```python
from build123d import *

# Parameters (mm, degrees)
F1_DEPTH = 5
F4_DEPTH = 2.54
F5_DEPTH = 25.4


with BuildPart() as f1:
    # F0 (on Front) → F1 (new body)
    with BuildSketch(Plane.XZ):
        with BuildLine():
            ThreePointArc((0, 20.9869445181), (-12.0966427586, 25.9236544676), (-24.1932855172, 20.9869445181))
            ThreePointArc((-24.1932855172, 20.9869445181), (-32.8877742223, 9.0834832543), (-21.2784307494, 0))
            ThreePointArc((-21.2784307494, 0), (-27.8345018972, -12.2317448258), (-21.2784307494, -24.4634896517))
            ThreePointArc((-21.2784307494, -24.4634896517), (-35.1701421662, -37.2707710413), (-38.4840406477, -55.8724962175))
            ThreePointArc((-38.4840406477, -55.8724962175), (-23.8469055846, -52.8720513548), (-9.2097705214, -55.8724962175))
            ThreePointArc((-9.2097705214, -55.8724962175), (-6.0029489911, -61.8966557159), (-2.7961274609, -55.8724962175))
            ThreePointArc((-2.7961274609, -55.8724962175), (9.7817579313, -54.6124723986), (22.2429726273, -56.7359104753))
            ThreePointArc((22.2429726273, -56.7359104753), (22.2759376745, -54.9746026101), (22.22623583, -53.2136875591))
            ThreePointArc((22.22623583, -53.2136875591), (18.366243738, -38.4713383456), (8.9641526372, -26.4781285077))
            ThreePointArc((8.9641526372, -26.4781285077), (9.8457214763, -18.7313808571), (8.9641526372, -10.9846332065))
            ThreePointArc((8.9641526372, -10.9846332065), (12.7377833841, 3.0446666193), (5.6262267365, 15.7130250237))
            Line((5.6262267365, 15.7130250237), (36.5616049228, 40.8807976003))
            ThreePointArc((36.5616049228, 40.8807976003), (34.4898748978, 53.7428757551), (23.25864156, 47.1410186325))
            Line((23.25864156, 47.1410186325), (0, 20.9869445181))
        make_face()
    extrude(amount=F1_DEPTH)

    # F5 (cut): a face of the model
    f5_faces = [f1.faces().sort_by_distance(p)[0] for p in [
        (-4.5967380367, -5, -11.98241047),
    ]]
    extrude(f5_faces, amount=-F5_DEPTH, mode=Mode.SUBTRACT)


with BuildPart() as f1b:
    # F0 (on Front) → F1, piece 2 (new body)
    with BuildSketch(Plane.XZ):
        with BuildLine():
            ThreePointArc((41.8436169818, -52.7066290379), (31.7747593943, -42.8946624715), (22.22623583, -53.2136875591))
            ThreePointArc((22.22623583, -53.2136875591), (32.2819872673, -62.5185956042), (41.8436169818, -52.7066290379))
        make_face()
    extrude(amount=F1_DEPTH)


with BuildPart() as f4:
    # F3 (on face) → F4 (new body)
    with BuildSketch(Plane.XZ.offset(5)):
        with BuildLine():
            ThreePointArc((-40.3169446951, -59.5749264298), (-26.5786982557, -55.5198668281), (-12.3739342893, -57.3658365623))
            ThreePointArc((-12.3739342893, -57.3658365623), (-6.2221601499, -64.4329037682), (0.3986158134, -57.8031911351))
            ThreePointArc((0.3986158134, -57.8031911351), (12.6136445695, -57.3475459696), (24.4946623983, -60.2208638043))
            ThreePointArc((24.4946623983, -60.2208638043), (22.3566756727, -41.3285471938), (11.7528280148, -25.5472598891))
            ThreePointArc((11.7528280148, -25.5472598891), (12.3852570181, -18.5459373039), (11.6827134618, -11.5513024358))
            ThreePointArc((11.6827134618, -11.5513024358), (15.3563975367, 2.4028081974), (9.5009837393, 15.5909577077))
            Line((9.5009837393, 15.5909577077), (38.2345170044, 38.9673983055))
            ThreePointArc((38.2345170044, 38.9673983055), (36.0298866682, 55.8114240261), (20.82786015, 48.229868306))
            Line((20.82786015, 48.229868306), (-0.2458838852, 24.5326862524))
            ThreePointArc((-0.2458838852, 24.5326862524), (-13.043561552, 28.4410317154), (-25.4100113891, 23.3296095701))
            ThreePointArc((-25.4100113891, 23.3296095701), (-35.5065684593, 11.3015480777), (-26.8662872673, -1.811814148))
            ThreePointArc((-26.8662872673, -1.811814148), (-30.3536378615, -13.0793756448), (-25.7757993219, -23.9496539557))
            ThreePointArc((-25.7757993219, -23.9496539557), (-38.9666786297, -39.3458023105), (-40.3169446951, -59.5749264298))
        make_face()
        with BuildLine():
            ThreePointArc((-2.7961274609, -55.8724962175), (-6.0029489911, -61.8966557159), (-9.2097705214, -55.8724962175))
            ThreePointArc((-9.2097705214, -55.8724962175), (-23.8469055846, -52.8720513548), (-38.4840406477, -55.8724962175))
            ThreePointArc((-38.4840406477, -55.8724962175), (-35.1701421662, -37.2707710413), (-21.2784307494, -24.4634896517))
            ThreePointArc((-21.2784307494, -24.4634896517), (-27.8345018972, -12.2317448258), (-21.2784307494, 0))
            ThreePointArc((-21.2784307494, 0), (-32.8877742223, 9.0834832543), (-24.1932855172, 20.9869445181))
            ThreePointArc((-24.1932855172, 20.9869445181), (-12.0966427586, 25.9236544676), (0, 20.9869445181))
            Line((0, 20.9869445181), (23.25864156, 47.1410186325))
            ThreePointArc((23.25864156, 47.1410186325), (34.4898748978, 53.7428757551), (36.5616049228, 40.8807976003))
            Line((36.5616049228, 40.8807976003), (5.6262267365, 15.7130250237))
            ThreePointArc((5.6262267365, 15.7130250237), (12.7377833841, 3.0446666193), (8.9641526372, -10.9846332065))
            ThreePointArc((8.9641526372, -10.9846332065), (9.8457214763, -18.7313808571), (8.9641526372, -26.4781285077))
            ThreePointArc((8.9641526372, -26.4781285077), (19.1118233272, -40.0673969806), (22.2429726273, -56.7359104753))
            ThreePointArc((22.2429726273, -56.7359104753), (9.7817579313, -54.6124723986), (-2.7961274609, -55.8724962175))
        make_face(mode=Mode.SUBTRACT)
    extrude(amount=F4_DEPTH)


solid = f4.part
```
Can you work these out from the model? Positions are in its coordinate system, mm. A direction names the side the tool comes from. Coordinates: 2 decimals unless noted, no trailing zeros. Order: outer loops, then holes, each group sorted by start corner. A loop starts at its lowest first (then second) coordinate and runs counter-clockwise, first axis right, second up.
1. Thinking about a two-plate mould opening in Z: for faces 3 (the face through (9.846, -6.252, -18.622)), 4 (the face through (12.44, -6.25, -57.33)), 5 (the face through (10.44, -6.25, 36.55)), 6 (the face through (12, -5, -8)), which applies, +Z half, -Z half, draft (parallel to the pull), parting line (faces both ways), or undercut?
2. If we section it at C-C (x = 19): Please give me the cut outline in (y, z), then the cut area to 3 significant figures.
3. I'm going to push flat-ended pins straight in: pin 1 (1 mm diameter, centred on y = -5.5, z = -27.5, fed in from +X); pin 2 (1 mm diameter, centred on x = -8.5, y = -5.5, fed in from -Z); pin 3 (1.5 mm diameter, centred on x = -24.5, y = -7, fed in from -Z). Where does each tip first touch, or does it pass through?
4. For faces 1 (the face through (-26.78, -6.252, -55.536)), 2 (the face through (-12.284, -6.252, 25.923)), which set-ups out of +Z, -Z, +X, -X, +Y, -Y let a thin tool reach every point of the face, with its end or its side?
5. If we section it at D-D (y = -5.5): Please give me the cut outline in (x, z), then the cut area to 3 significant figures.
6. I need wall thicknesses on line 1 (Z direction, x = 13.5, y = -6.5); line 2 (Z direction, x = -22.5, y = -7.35); line 3 (Z direction, x = 15.5, y = -6.6). Which ranges of each line are inside material? Lowest first, please.
7. If we section it at A-A (z = -37): Please give me the cut outline in (x, y).
8. If we section it at B-B (x = 30): Please give me the cut outline in (y, z).
Entries:
1. face 3: undercut
1. face 4: -Z half
1. face 5: +Z half
1. face 6: draft
2. outline: (-7.54, -58.46) - (-5, -58.46) - (-5, -55.85) - (-7.54, -55.85) - close; (-7.54, -39.82) - (-5, -39.82) - (-5, -34.36) - (-7.54, -34.36) - close; (-7.54, 23.32) - (-5, 23.32) - (-5, 26.59) - (-7.54, 26.59) - close; (-7.54, 42.35) - (-5, 42.35) - (-5, 46.17) - (-7.54, 46.17) - close
2. area: 38.5 mm2
3. pin 1: stops at x = 14.22
3. pin 2: stops at z = -64.12
3. pin 3: stops at z = -55.44
4. face 1: -Z, +Y, -Y
4. face 2: +Y, -Y
5. outline: (-40.32, -59.57) arc R34.66 cw to (-12.37, -57.37) arc R6.41 ccw (long way) to (0.4, -57.8) arc R44.66 cw to (24.49, -60.22) arc R40.08 ccw to (11.75, -25.55) arc R37.02 ccw to (11.68, -11.55) arc R21.78 ccw to (9.5, 15.59) - (38.23, 38.97) arc R10.43 ccw (long way) to (20.83, 48.23) - (-0.25, 24.53) arc R19.83 ccw to (-25.41, 23.33) arc R13.14 ccw to (-26.87, -1.81) arc R17.23 ccw to (-25.78, -23.95) arc R32.14 ccw to start; hole (-38.48, -55.87) arc R37.2 cw to (-9.21, -55.87) arc R3.87 ccw (long way) to (-2.8, -55.87) arc R47.2 cw to (22.24, -56.74) arc R37.54 ccw to (8.96, -26.48) arc R34.48 ccw to (8.96, -10.98) arc R19.24 ccw to (5.63, 15.71) - (36.56, 40.88) arc R7.89 ccw (long way) to (23.26, 47.14) - (0, 20.99) arc R17.29 ccw to (-24.19, 20.99) arc R10.6 ccw to (-21.28, 0) arc R14.69 ccw to (-21.28, -24.46) arc R29.6 ccw to start
5. area: 981 mm2
6. line 1: z = -57.45 to -54.89, -31.03 to -27.24, -8.3 to 9.61, 18.84 to 22.12, 36.17 to 39.99
6. line 2: z = -55.44 to -52.9, -25.04 to -23.56, -0.91 to -0.06, 22.44 to 25.52
6. line 3: z = -57.73 to -55.16, -33.64 to -29.46, 20.47 to 23.75, 38.42 to 42.24
7. outline: (-37.9, -7.54) - (-35.02, -7.54) - (-35.02, -5) - (-37.9, -5) - close; (17.6, -7.54) - (20.47, -7.54) - (20.47, -5) - (17.6, -5) - close
8. outline: (-7.54, 32.27) - (-5, 32.27) - (-5, 35.54) - (-7.54, 35.54) - close; (-7.54, 54.41) - (-5, 54.41) - (-5, 56.97) - (-7.54, 56.97) - close
